For this review, take the finished solid that the model builds, in its own axes (mm). A direction names the side the tool comes from. Coordinates: 2 decimals unless noted, no trailing zeros. Write each loop counter-clockwise with the first axis right and the second up, starting at its lowest first coordinate (ties: lowest second). Pieces come first, ordered by that corner, then holes. Notation, with made-up numbers: M 51.5,-19.75 L 91.5,-19.75 A32 ccw 91.5,13.25 Z; hole C 76.25,53.5 d5. An arc over 180 degrees is marked long. One line per question, with ' | ' between items.
from build123d import *

# Parameters (mm, degrees)
BOSS_EXTRUDE1_DEPTH = 825.5
FILLET1_R           = 1.27


with BuildPart() as part:
    # Sketch1 → Boss-Extrude1 (new body)
    with BuildSketch(Plane.XY):
        Polygon((0, 12.7), (-14.2875, 12.7), (-14.2875, 0), (-35.71875, 0), (-35.71875, 21.43125), (-23.01875, 21.43125), (-23.01875, 61.11875), (-35.71875, 61.11875), (-35.71875, 82.55), (-14.2875, 82.55), (-14.2875, 69.85), (0, 69.85), (0, 68.58), (-15.5575, 68.58), (-15.5575, 81.28), (-34.44875, 81.28), (-34.44875, 62.38875), (-21.74875, 62.38875), (-21.74875, 20.16125), (-34.44875, 20.16125), (-34.44875, 1.27), (-15.5575, 1.27), (-15.5575, 13.97), (0, 13.97), align=None)
    extrude(amount=-BOSS_EXTRUDE1_DEPTH)

    # Fillet1
    fillet1_edges = [part.edges().sort_by_distance(p)[0] for p in [
        (-14.2875, 0, -412.75),
        (-35.71875, 0, -412.75),
        (-35.71875, 21.43125, -412.75),
        (-35.71875, 61.11875, -412.75),
        (-35.71875, 82.55, -412.75),
        (-14.2875, 82.55, -412.75),
        (-15.5575, 68.58, -412.75),
        (-21.74875, 62.38875, -412.75),
        (-21.74875, 20.16125, -412.75),
        (-15.5575, 13.97, -412.75),
    ]]
    fillet(fillet1_edges, radius=FILLET1_R)


solid = part.part
1) To check wall thickness, follow line 1 along Y through (x, z) = (-26, -262); line 2 along Y through (x, z) = (-9.5, -58.5); line 3 along X through (y, z) = (71.5, -186.5). State the ranges of each line that lie inside material, in increasing order. Write a range as [from, to].
Responses:
line 1: [0, 1.27], [20.16, 21.43], [61.12, 62.39], [81.28, 82.55] | line 2: [12.7, 13.97], [68.58, 69.85] | line 3: [-35.72, -34.45], [-15.56, -14.29]
2) Machinability: for faces 4 (the flat face through (-7, 68.58, -407)), 5 (the flat face through (-7, 69.85, -407)), 6 (the flat face through (-34.449, 72, -407)), which of the approach directions +Z, -Z, +X, -X, +Y, -Y give a long, thin tool a straight path to every point of the face, cutting with its end or side? Answer none if there is none.
Responses:
face 4: +Z, -Z, +X | face 5: +Z, -Z, +X, +Y | face 6: +Z, -Z
3) We need section B-B on y = 39.5. State the section outline as (x, z) points.
Responses:
outline: M -23.02,-825.5 L -21.75,-825.5 L -21.75,0 L -23.02,0 Z
4) The part is to be moulded in two halves that separate along X. For faces 1 (the flat face through (-25, 81.28, -407)), 2 (the flat face through (-35.719, 11, -407)), 3 (the flat face through (-7, 12.7, -407)), say which applies: +X half, -X half, draft (parallel to the pull), parting line (faces both ways), or undercut.
Responses:
face 1: undercut | face 2: -X half | face 3: draft
5) Insertion check: pin 1 Ø12 at (y, z) = (37, -716.5) entering from +X; pin 2 Ø6 at (x, z) = (-4.5, -495.5) entering from +Y; pin 3 Ø9 at (y, z) = (76.5, -418) entering from +X; pin 4 Ø12 at (x, y) = (-28.5, 45) entering from +Z. Each pin has a flat end and moves straight along its axis. Give the tip position at first contact, or say it passes through.
Responses:
pin 1: x = -21.75 | pin 2: y = 69.85 | pin 3: x = -14.29 | pin 4: z = 0
